Geometry: see drawing. Coordinates: mm, zero at the bounding-box minimum. A direction names the side the tool comes from. Give positions to 0.01 mm unless a question says otherwise; leave off trailing zeros. Write each loop counter-clockwise with the first axis right and the second up, starting at its lowest first coordinate (ties: lowest second). Pieces come first, ordered by that corner, then holes. Notation, with made-up numbers: M -19,-1 L 12,-1 A15 ccw 12,24 Z; hole C 10.5,20.25 d6. An arc over 180 degrees is marked long. Use a Markdown table: item, result. Add a question column.
1) Section A-A on x = 6.35. Return the cut outline in (y, z) (1 decimal), then the cut area to 3 significant figures.
2) Section B-B on z = 15.5. Return the cut outline in (x, y).
3) Pin query (flat end, axial travel): pin 1 (4 mm diameter, centred on y = 4, z = 6, fed in from -X); pin 2 (3 mm diameter, centred on x = 9.5, z = 5, fed in from +Y) (1 decimal); pin 3 (1 mm diameter, centred on x = 6.5, z = 24, fed in from -Y). Return the tip coordinate at first contact, or that it passes through.
4) Set-up query: the marked faces 1 and 2. Return all of +Z, -Z, +X, -X, +Y, -Y with unobstructed straight access to the full face (end or side cutting, diameter ignored); none if empty.
5) Line query: line 1 (X direction, y = 6.5, z = 26.5); line 2 (Z direction, x = 8, y = 2.75) (1 decimal). Output: solid intervals per line, ascending.
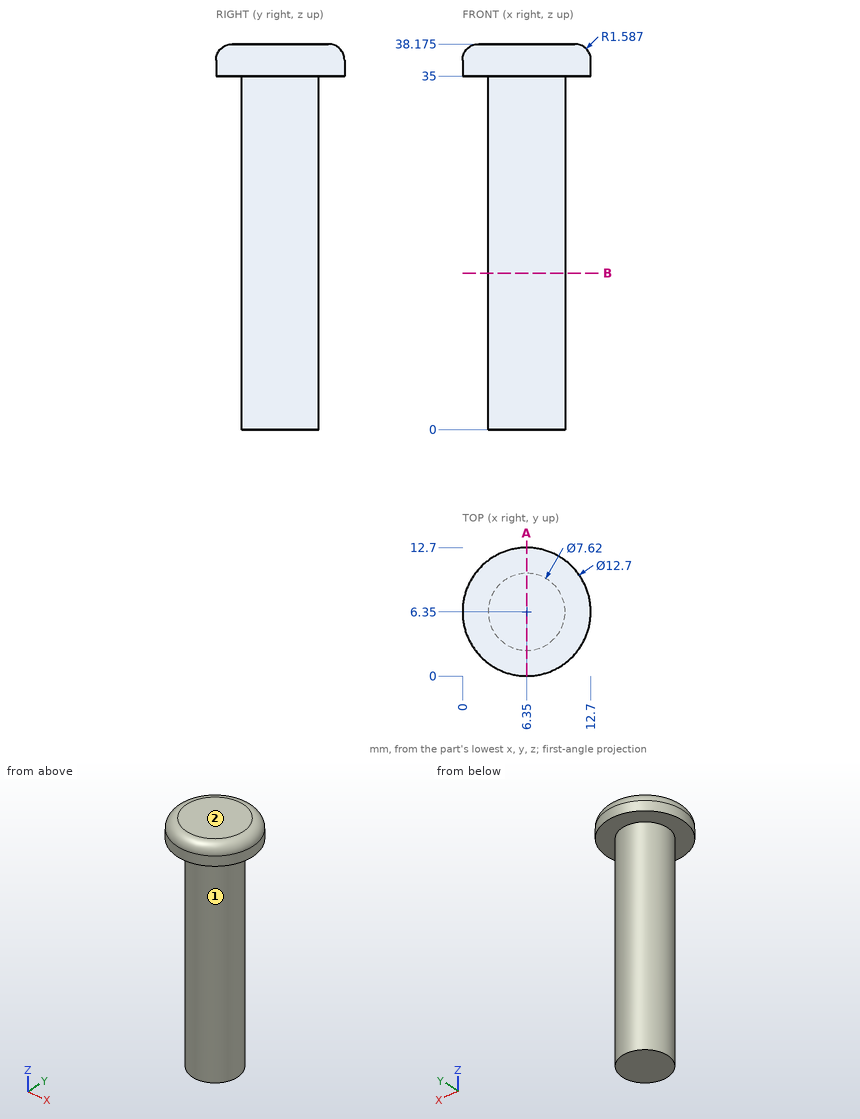
Found:
| question | item | result |
|---|---|---|
| 1 | outline | M 0,35 L 2.5,35 L 2.5,0 L 10.2,0 L 10.2,35 L 12.7,35 L 12.7,36.6 A1.6 ccw 11.1,38.2 L 1.6,38.2 A1.6 ccw 0,36.6 Z |
| 1 | area | 306 mm² |
| 2 | outline | C 6.35,6.35 d7.62 |
| 3 | pin 1 | x = 2.56 |
| 3 | pin 2 | y = 9.8 |
| 3 | pin 3 | y = 2.54 |
| 4 | face 1 | -Z |
| 4 | face 2 | +Z, +X, -X, +Y, -Y |
| 5 | line 1 | 2.54 to 10.16 |
| 5 | line 2 | 35 to 38.2 |
